Autodesk Inventor part; units mm, degrees
ref_plane "YZ Plane" through (0, 0, 0) normal (1, 0, 0) x (0, 1, 0)
ref_plane "XZ Plane" through (0, 0, 0) normal (0, 1, 0) x (-1, 0, 0)
ref_plane "XY Plane" through (0, 0, 0) normal (0, 0, 1) x (1, 0, 0)
sketch "Sketch1" plane through (0, 0, 0) normal (0, 1, 0) x (-1, 0, 0)
  circle A0 centre (0, 0) radius 10.25
  circle A1 centre (0, 0) radius 3
  line L0 (0, 0) -> (0, 7.25)
  line L1 (0, 0) -> (-4.2614, 5.8654)
  line L2 (0, 0) -> (-6.8952, 2.2404)
  line L3 (0, 0) -> (-6.8952, -2.2404)
  line L4 (0, 0) -> (-4.2614, -5.8654)
  line L5 (0, 0) -> (0, -7.25)
  line L6 (0, 0) -> (4.2614, -5.8654)
  line L7 (0, 0) -> (6.8952, -2.2404)
  line L8 (0, 0) -> (6.8952, 2.2404)
  line L9 (0, 0) -> (4.2614, 5.8654)
  arc A2 (4.2614, 5.8654) -> (0, 7.25) centre (0, 0) ccw
  arc A3 (-4.2614, 5.8654) -> (-6.8952, 2.2404) centre (0, 0) ccw
  arc A4 (-6.8952, -2.2404) -> (-4.2614, -5.8654) centre (0, 0) ccw
  arc A5 (0, -7.25) -> (4.2614, -5.8654) centre (0, 0) ccw
  arc A6 (6.8952, -2.2404) -> (6.8952, 2.2404) centre (0, 0) ccw
  arc A7 (4.2614, 5.8654) -> (0, 7.25) centre (0, 0) ccw
  arc A8 (6.8952, -2.2404) -> (6.8952, 2.2404) centre (0, 0) ccw
  arc A9 (0, -7.25) -> (4.2614, -5.8654) centre (0, 0) ccw
  arc A10 (-6.8952, -2.2404) -> (-4.2614, -5.8654) centre (0, 0) ccw
  arc A11 (-4.2614, 5.8654) -> (-6.8952, 2.2404) centre (0, 0) ccw
  circle A12 centre (0, 0) radius 3
  dimension "d0" = 20.5
  dimension "d2" = 6
  dimension "d5" = 360
extrude "Extrusion1" add sketch "Sketch1" along normal blind 10 contours A0 | A1 L7 L8 | A1 L8 A6 L7 | L8 L9 A1 | A1 L6 L7 | L9 L0 A1 | A1 L0 A2 L9 | L1 A1 L0 | L2 A1 L1 | L3 A1 L2 | L4 A1 L3 | L5 A1 L4 | L6 A1 L5 | L6 A5 L5 A1 | A1 L2 A3 L1
sketch "Sketch2" plane through (0, 10, 0) normal (0, 1, 0) x (1, 0, 0)
  point P0 (0, 0)
sketch "Sketch3" plane through (0, 10, 0) normal (0, 1, 0) x (1, 0, 0)
  arc A0 (2.8532, 0.9271) -> (1.7634, 2.4271) centre (0, 0) ccw
  line L0 (1.7634, 2.4271) -> (4.2614, 5.8654)
  arc A1 (6.8952, 2.2404) -> (4.2614, 5.8654) centre (0, 0) ccw
  line L1 (6.8952, 2.2404) -> (2.8532, 0.9271)
  line L2 (-1.2202, 2.7406) -> (-2.9488, 6.6232)
  arc A2 (0.6237, 2.9344) -> (-1.2202, 2.7406) centre (0, 0) ccw
  line L3 (1.5074, 7.0916) -> (0.6237, 2.9344)
  arc A3 (1.5074, 7.0916) -> (-2.9488, 6.6232) centre (0, 0) ccw
  line L4 (-2.9836, 0.3136) -> (-7.2103, 0.7578)
  arc A4 (-2.2294, 2.0074) -> (-2.9836, 0.3136) centre (0, 0) ccw
  line L5 (-5.3878, 4.8512) -> (-2.2294, 2.0074)
  arc A5 (-5.3878, 4.8512) -> (-7.2103, 0.7578) centre (0, 0) ccw
  line L6 (-1.7634, -2.4271) -> (-4.2614, -5.8654)
  arc A6 (-2.8532, -0.9271) -> (-1.7634, -2.4271) centre (0, 0) ccw
  line L7 (-6.8952, -2.2404) -> (-2.8532, -0.9271)
  arc A7 (-6.8952, -2.2404) -> (-4.2614, -5.8654) centre (0, 0) ccw
  line L8 (1.2202, -2.7406) -> (2.9488, -6.6232)
  arc A8 (-0.6237, -2.9344) -> (1.2202, -2.7406) centre (0, 0) ccw
  line L9 (-1.5074, -7.0916) -> (-0.6237, -2.9344)
  arc A9 (-1.5074, -7.0916) -> (2.9488, -6.6232) centre (0, 0) ccw
  line L10 (2.9836, -0.3136) -> (7.2103, -0.7578)
  arc A10 (2.2294, -2.0074) -> (2.9836, -0.3136) centre (0, 0) ccw
  line L11 (5.3878, -4.8512) -> (2.2294, -2.0074)
  arc A11 (5.3878, -4.8512) -> (7.2103, -0.7578) centre (0, 0) ccw
  dimension "d11" = 360
extrude "Extrusion2" cut sketch "Sketch3" against normal blind 10 contours L2 A3 L3 A2 | L4 A5 L5 A4 | L6 A7 L7 A6 | L8 A9 L9 A8 | L10 A11 L11 A10
fillet "Fillet1" radius 1 21 edges at (-6.8952, 5, 2.2404) (-7.2103, 5, -0.7578) (-2.9488, 5, -6.6232) (1.7634, 5, -2.4271) (2.2294, 5, 2.0074) (-1.5074, 5, 7.0916) (2.8532, 5, -0.9271) (2.9488, 5, 6.6232) (-2.9836, 5, -0.3136) (6.8952, 5, -2.2404) (5.3878, 5, 4.8512) (7.2103, 5, 0.7578) (1.5074, 5, -7.0916) (-5.3878, 5, -4.8512) (4.2614, 5, -5.8654) (-0.6237, 5, 2.9344) (1.2202, 5, 2.7406) (-2.8532, 5, 0.9271) (-4.2614, 5, 5.8654) (-1.7634, 5, 2.4271) (-2.2294, 5, -2.0074)
sketch "Sketch4" plane through (0, 10, 0) normal (0, 1, 0) x (1, 0, 0)
  circle A0 centre (0, 0) radius 1.5
  dimension "d16" = 3
extrude "Extrusion3" cut sketch "Sketch4" against normal blind 10
properties part number "rin"
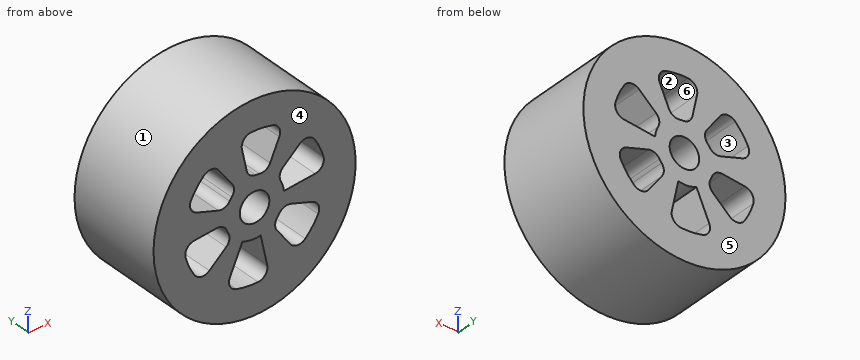
Can you work these out from the model? Positions are in its coordinate system, mm. Face numbers are marked on the shaded views. A direction names the side the tool comes from. Give positions to 0.01 mm unless a question says otherwise; leave off trailing zeros. Order: outer loops, then holes, each group sorted by start corner. A loop starts at its lowest first (then second) coordinate and runs counter-clockwise, first axis right, second up. Notation, with made-up numbers: M 73.25,12 L 89.25,12 A38 cw 89.25,50 Z; hole C 13,79.25 d1. An arc over 180 degrees is marked long. Write item = value, one per line. Start each with the question number.
Q1. I need wall thicknesses on probe 1 along Z at (x, y) = (0, 3.25); probe 2 along X at (y, z) = (2.75, -3.5); probe 3 along Z at (x, y) = (-0.5, 0.75). Which ranges of each line are inside material? Lowest first, please. Write a range as [from, to].
Q2. Suppose I cut it at B-B (y = 7.5). Count the separate pieces of the cut face and the enclosed holes in it, plus the area to 3 significant figures.
Q3. Suppose I cut it at C-C (z = -8.5). Write out the boundary of the cut face in (x, y), plus the area to 3 significant figures.
Q4. Will these pins go through, and if not, where does the flat tip stop? pin 1 Ø1.5 at (y, z) = (3, 5.5) entering from -X; pin 2 Ø6 at (y, z) = (2, 8) entering from -X; pin 3 Ø2 at (x, y) = (-8, 5.5) entering from +Z.
Q5. For the marked faces 5 and 6, which set-ups out of +Z, -Z, +X, -X, +Y, -Y let a thin tool reach every point of the face, with its end or its side?
Q6. Suppose I cut it at A-A (z = 0). Write out the boundary of the cut face in (x, y), plus the area to 3 significant figures.
Q7. We'd pull the mould along Z, two halves only. Please class the marked faces 1, 2, 3 and 4: pulls with the +Z half, pulls with the -Z half, needs draft (parallel to the pull), parting line crosses it, or undercut.
Check result:
q1.probe_1 = [-10.25, -7.25], [-3, -1.5], [1.5, 3.01], [7.25, 10.25]
q1.probe_2 = [-9.63, -6.35], [-3.89, -1.56], [0.74, 2.54], [6.35, 9.63]
q1.probe_3 = [-10.24, -7.23], [-2.96, -1.41], [1.41, 3.26], [7.22, 10.24]
q2.separate_pieces = 1
q2.enclosed_holes = 7
q2.area = 245 mm2
q3.outline = M -5.73,0 L 5.73,0 L 5.73,10 L -5.73,10 Z
q3.area = 115 mm2
q4.pin_1 = -9.08
q4.pin_2 = -8.95
q4.pin_3 = 7.49
q5.face_5 = +Z, -Z, +X, -X, +Y
q5.face_6 = +Y, -Y
q6.outline = M -10.25,0 L -1.5,0 L -1.5,10 L -10.25,10 Z; M 1.5,0 L 10.25,0 L 10.25,10 L 1.5,10 Z
q6.area = 175 mm2
q7.face_1 = parting line crosses it
q7.face_2 = undercut
q7.face_3 = undercut
q7.face_4 = needs draft
